Could you check a few things on this model? Use its own coordinates, in mm. Coordinates: 2 decimals unless noted, no trailing zeros. Write each loop counter-clockwise with the first axis right and the second up, starting at its lowest first coordinate (ties: lowest second). Pieces come first, ordered by that corner, then holes. Notation, with made-up numbers: M 29,-11.75 L 33,-11.75 A13 cw 33,-7.75 Z; hole C 60.25,9.25 d3. An arc over 180 degrees is marked long. Answer as CSV lines item,"result". Start each with the question number.
Item 1: I'm going to push a flat-ended pin straight in: P1, Ø3, axis at x = 5.5, y = -42, coming from the +Z side. Where does the tip first touch, or does it pass through?
Item 2: Suppose I cut it at A-A, the plane x = 80. Write out the boundary of the cut face in (y, z).
Item 3: If I drill on line 1 along X through (y, z) = (-40.75, 13.5); line 2 along Y through (x, z) = (80, 30.5); line 3 along Y through (x, z) = (66.5, 47), over which ranges is the centre line in solid material (lowest first)? Write a range as [from, to].
Item 4: Suppose I cut it at B-B, the plane y = -38.75. Write out the boundary of the cut face in (x, z).
Item 5: Suppose I cut it at C-C, the plane z = 28. State how many separate pieces and enclosed holes the cut face has, and give its area (3 significant figures).
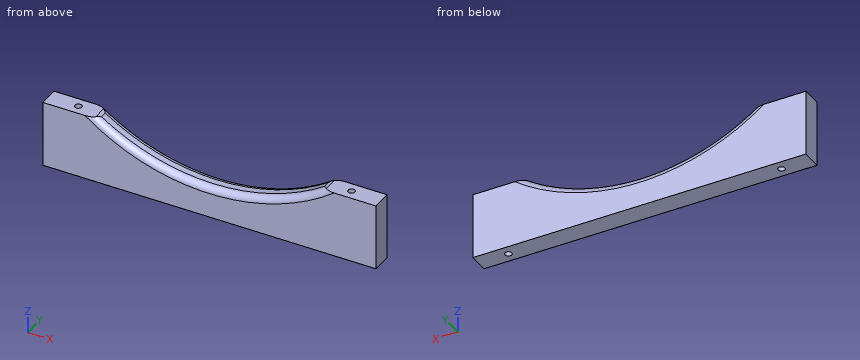
```python
from build123d import *

# Parameters (mm, degrees)
SKETCH1_R           = 2.5
BOSS_EXTRUDE1_DEPTH = 50
CUT_EXTRUDE1_DEPTH  = 15
FILLET1_R           = 5


with BuildPart() as part:
    # Sketch1 → Boss-Extrude1 (new body)
    with BuildSketch(Plane.XY):
        Polygon((80, -46.25), (102.5, -46.25), (102.5, -31.25), (80, -31.25), (-147.5, -31.25), (-147.5, -46.25), align=None)
        with Locations((-125, -38.75)):
            Circle(SKETCH1_R, mode=Mode.SUBTRACT)
        with Locations((80, -38.75)):
            Circle(SKETCH1_R, mode=Mode.SUBTRACT)
    extrude(amount=BOSS_EXTRUDE1_DEPTH)

    # Sketch2 → Cut-Extrude1 (cut)
    with BuildSketch(Plane.XZ.offset(46.25)):
        with BuildLine():
            Line((-107.5, 50), (62.5, 50))
            ThreePointArc((62.5, 50), (-22.5, 23.592070943), (-107.5, 50))
        make_face()
    extrude(amount=-CUT_EXTRUDE1_DEPTH, mode=Mode.SUBTRACT)

    # Fillet1
    fillet1_edges = [part.edges().sort_by_distance(p)[0] for p in [
        (62.5, -38.75, 50),
        (-107.5, -38.75, 50),
        (-22.5, -46.25, 23.592070943),
        (-22.5, -31.25, 23.592070943),
    ]]
    fillet(fillet1_edges, radius=FILLET1_R)


solid = part.part
```
Ans:
1,P1,"stops at z = 26.5"
2,outline,"M -46.25,0 L -41.25,0 L -41.25,50 L -46.25,50 Z; M -36.25,0 L -31.25,0 L -31.25,50 L -36.25,50 Z"
3,line 1,"x = [-147.5, -126.5], [-123.5, 78.5], [81.5, 102.5]"
3,line 2,"y = [-46.25, -41.25], [-36.25, -31.25]"
3,line 3,"y = [-46.24, -31.26]"
4,outline,"M -147.5,0 L -127.5,0 L -127.5,50 L -147.5,50 Z; M -122.5,0 L 77.5,0 L 77.5,50 L 64.04,50 A5 ccw 61.25,49.15 A150 cw -106.25,49.15 A5 ccw -109.04,50 L -122.5,50 Z; M 82.5,0 L 102.5,0 L 102.5,50 L 82.5,50 Z"
5,separate pieces,"2"
5,enclosed holes,"2"
5,area,"2,550 mm^2"
